Source: CAD feature listing. Evaluate the final solid. Frame: model axes, mm. A direction names the side the tool comes from. Coordinates: 2 decimals unless noted, no trailing zeros. Order: outer loops, then holes, each group sorted by start corner. A loop starts at its lowest first (then second) coordinate and runs counter-clockwise, first axis right, second up.
```python
from build123d import *
from build123d.topology import SkipClean

# Parameters (mm, degrees)
SKETCH1_R               = 10
BOSS_EXTRUDE1_DEPTH     = 15
CUT_EXTRUDE1_DEPTH      = 10
BOSS_EXTRUDE2_DEPTH     = 10
CUT_EXTRUDE2_DEPTH      = 184.098334236
CUT_EXTRUDE2_DEPTH_BACK = 184.098334236


with BuildPart() as part:
    # Sketch1 → Boss-Extrude1 (new, symmetric)
    with BuildSketch(Plane.XY):
        with BuildLine():
            ThreePointArc((24.881082953, -2.435510432), (0, 25), (-24.881082953, -2.435510432))
            Line((-24.881082953, -2.435510432), (-7.5, -180))
            Line((-7.5, -180), (7.5, -180))
            Line((7.5, -180), (24.881082953, -2.435510432))
        make_face()
        Circle(SKETCH1_R, mode=Mode.SUBTRACT)
    extrude(amount=BOSS_EXTRUDE1_DEPTH, both=True)

    # Sketch1_4 → Cut-Extrude1 (cut, symmetric)
    with SkipClean():  # the faces are left unmerged after this step: merging them gives an invalid solid
        with BuildSketch(Plane.XY):
            with BuildLine():
                ThreePointArc((30, 0), (28.266291258, -10.05071035), (23.265548098, -18.939753739))
                Line((23.265548098, -18.939753739), (22.15809951, -30.253406851))
                ThreePointArc((22.15809951, -30.253406851), (33.445319042, -16.96056114), (37.5, 0))
                ThreePointArc((37.5, 0), (-16.96056114, 33.445319042), (-22.15809951, -30.253406851))
                Line((-22.15809951, -30.253406851), (-23.265548098, -18.939753739))
                ThreePointArc((-23.265548098, -18.939753739), (-10.05071035, 28.266291258), (30, 0))
            make_face()
            with BuildLine():
                Line((22.15809951, -30.253406851), (23.265548098, -18.939753739))
                ThreePointArc((23.265548098, -18.939753739), (0, -30), (-23.265548098, -18.939753739))
                Line((-23.265548098, -18.939753739), (-22.15809951, -30.253406851))
                ThreePointArc((-22.15809951, -30.253406851), (0, -37.5), (22.15809951, -30.253406851))
            make_face()
            with BuildLine():
                ThreePointArc((25, 0), (24.970253041, -1.219205923), (24.881082953, -2.435510432))
                Line((24.881082953, -2.435510432), (23.265548098, -18.939753739))
                ThreePointArc((23.265548098, -18.939753739), (28.266291258, -10.05071035), (30, 0))
                ThreePointArc((30, 0), (-10.05071035, 28.266291258), (-23.265548098, -18.939753739))
                Line((-23.265548098, -18.939753739), (-24.881082953, -2.435510432))
                ThreePointArc((-24.881082953, -2.435510432), (-1.219205923, 24.970253041), (25, 0))
            make_face()
            with BuildLine():
                Line((23.265548098, -18.939753739), (24.881082953, -2.435510432))
                ThreePointArc((24.881082953, -2.435510432), (0, -25), (-24.881082953, -2.435510432))
                Line((-24.881082953, -2.435510432), (-23.265548098, -18.939753739))
                ThreePointArc((-23.265548098, -18.939753739), (0, -30), (23.265548098, -18.939753739))
            make_face()
        extrude(amount=CUT_EXTRUDE1_DEPTH, both=True, mode=Mode.SUBTRACT)

    # Sketch1_5 → Boss-Extrude2 (add, symmetric)
    with BuildSketch(Plane.XY):
        with BuildLine():
            ThreePointArc((25, 0), (24.970253041, -1.219205923), (24.881082953, -2.435510432))
            Line((24.881082953, -2.435510432), (23.265548098, -18.939753739))
            ThreePointArc((23.265548098, -18.939753739), (28.266291258, -10.05071035), (30, 0))
            ThreePointArc((30, 0), (-10.05071035, 28.266291258), (-23.265548098, -18.939753739))
            Line((-23.265548098, -18.939753739), (-24.881082953, -2.435510432))
            ThreePointArc((-24.881082953, -2.435510432), (-1.219205923, 24.970253041), (25, 0))
        make_face()
        with BuildLine():
            Line((23.265548098, -18.939753739), (24.881082953, -2.435510432))
            ThreePointArc((24.881082953, -2.435510432), (0, -25), (-24.881082953, -2.435510432))
            Line((-24.881082953, -2.435510432), (-23.265548098, -18.939753739))
            ThreePointArc((-23.265548098, -18.939753739), (0, -30), (23.265548098, -18.939753739))
        make_face()
    extrude(amount=BOSS_EXTRUDE2_DEPTH, both=True)

    # Sketch3 → Cut-Extrude2 (cut, two sides: drawn at the far end of the back side and taken through both)
    with BuildSketch(Plane(origin=(0, 0, 0), x_dir=(0, 0, -1), z_dir=(1, 0, 0)).offset(-CUT_EXTRUDE2_DEPTH_BACK)):
        Polygon((-15, -180), (-7.5, -180), (-15, -40), align=None)
        Polygon((15, -40), (7.5, -180), (15, -180), align=None)
    extrude(amount=CUT_EXTRUDE2_DEPTH + CUT_EXTRUDE2_DEPTH_BACK, mode=Mode.SUBTRACT)


solid = part.part
```
1. Contact query for flat-ended pins moving along their axis: P1, Ø6, axis at y = -144.5, z = 7, coming from the +X side; P2, Ø4, axis at x = 13, z = -8.5, coming from the +Y side; P3, Ø1, axis at y = -118, z = -7.5, coming from the +X side; P4, Ø12, axis at x = 0, y = 0, coming from the +Z side. Output: stop coordinate, or through.
2. Section query B-B, the plane z = 4. Output: boundary loops of the cut face in (x, y), plus the area to 3 significant figures.
3. Access query for faces 1 (the flat face through (-0.3, -30.2, 10)), 2 (the flat face through (0, -180, 0)). Directions: +Z, -Z, +X, -X, +Y, -Y. A direction counts if a zero-diameter tool reaches every point of the face in a straight line with its end or side. Return the directions, or none.
4. Section query C-C, the plane z = -12. Output: boundary loops of the cut face in (x, y), plus the area to 3 significant figures.
5. Section query A-A, the plane x = 0. Output: boundary loops of the cut face in (y, z), plus the area to 3 significant figures.
6. Material intervals for line 1 along Y through (x, z) = (0, -2.5); line 2 along Y through (x, z) = (4, -3.75); line 3 along Z through (x, y) = (-26, -13), sorted ascending.
7. Section query D-D, the plane y = -137. Output: boundary loops of the cut face in (x, z), plus the area to 3 significant figures.
8. Draft query along Y for faces 3 (the cylindrical face through (-2.17, -9.76, -0.21)), 4 (the flat face through (0, -14, 15)), 5 (the flat face through (-0.3, -95.42, 12.03)), 6 (the flat face through (-0.3, -30.2, -10)). Return one class per face: +Y half, -Y half, draft (parallel to the pull), parting line (faces both ways), or undercut.
Answer key:
1. P1: stops at x = 11.27
1. P2: stops at y = 27.91
1. P3: stops at x = 13.62
1. P4: passes through
2. outline: circle Ø60 at (0, 0); (-22.16, -30.25) - (-7.5, -180) - (7.5, -180) - (22.16, -30.25) arc R37.5 cw to start; hole circle Ø20 at (0, 0)
2. area: 6,740 mm2
3. face 1: none
3. face 2: +Z, -Z, +X, -X, -Y
4. outline: (-24.88, -2.44) - (-15.72, -96) - (15.72, -96) - (24.88, -2.44) arc R25 ccw (long way) to start; hole circle Ø20 at (0, 0)
4. area: 4,590 mm2
5. outline: (-180, -7.5) - (-40, -15) - (-10, -15) - (-10, 15) - (-40, 15) - (-180, 7.5) - close; (10, -15) - (25, -15) - (25, -10) - (30, -10) - (30, 10) - (25, 10) - (25, 15) - (10, 15) - close; hole (-37.5, -10) - (-30, -10) - (-30, 10) - (-37.5, 10) - close
5. area: 4,450 mm2
6. line 1: y = -180 to -37.5, -30 to -10, 10 to 30
6. line 2: y = -180 to -37.29, -29.73 to -9.17, 9.17 to 29.73
6. line 3: z = -10 to 10
7. outline: (-11.71, -9.8) - (11.71, -9.8) - (11.71, 9.8) - (-11.71, 9.8) - close
7. area: 459 mm2
8. face 3: undercut
8. face 4: draft
8. face 5: -Y half
8. face 6: undercut
